Design review of the part shown in the three views and the two pictorial views. Dimensions are in mm from the part's minimum x, y and z. A direction names the side the tool comes from. Give positions to 0.01 mm unless a question says otherwise; leave off trailing zeros. Order: outer loops, then holes, each group sorted by start corner. A loop starts at its lowest first (then second) coordinate and runs counter-clockwise, first axis right, second up.
Item 1: The part is to be moulded in two halves that separate along X. For the marked faces 1, 2 and 3, say which applies: released by +X, released by -X, zero draft, split by the parting line, or undercut.
Item 2: For P1, Ø1.5, axis at x = 14, z = 1, coming from the +Y side, flat-tipped, find the tip position at first contact; note if it passes through.
Item 3: Machinability: for the marked faces 4, 5 and 6, which of the approach directions +Z, -Z, +X, -X, +Y, -Y give a long, thin tool a straight path to every point of the face, cutting with its end or side? Answer none if there is none.
Item 4: Consider section D-D (y = 7.75). Give the boundary of the cut face in (x, z), plus the area to 3 significant figures.
Item 5: Consider section A-A (y = 16.5). Give the boundary of the cut face in (x, z), plus the area to 3 significant figures.
Item 6: Consider section B-B (x = 7.6). Give the boundary of the cut face in (y, z), plus the area to 3 significant figures.
Item 7: For probe 1 along Y at (x, z) = (7.6, 0.95); probe 2 along X at (y, z) = (10.5, 0.85); probe 3 along Y at (x, z) = (14, 2.65), list the stretches that pass through material, from the lowest coordinate up.
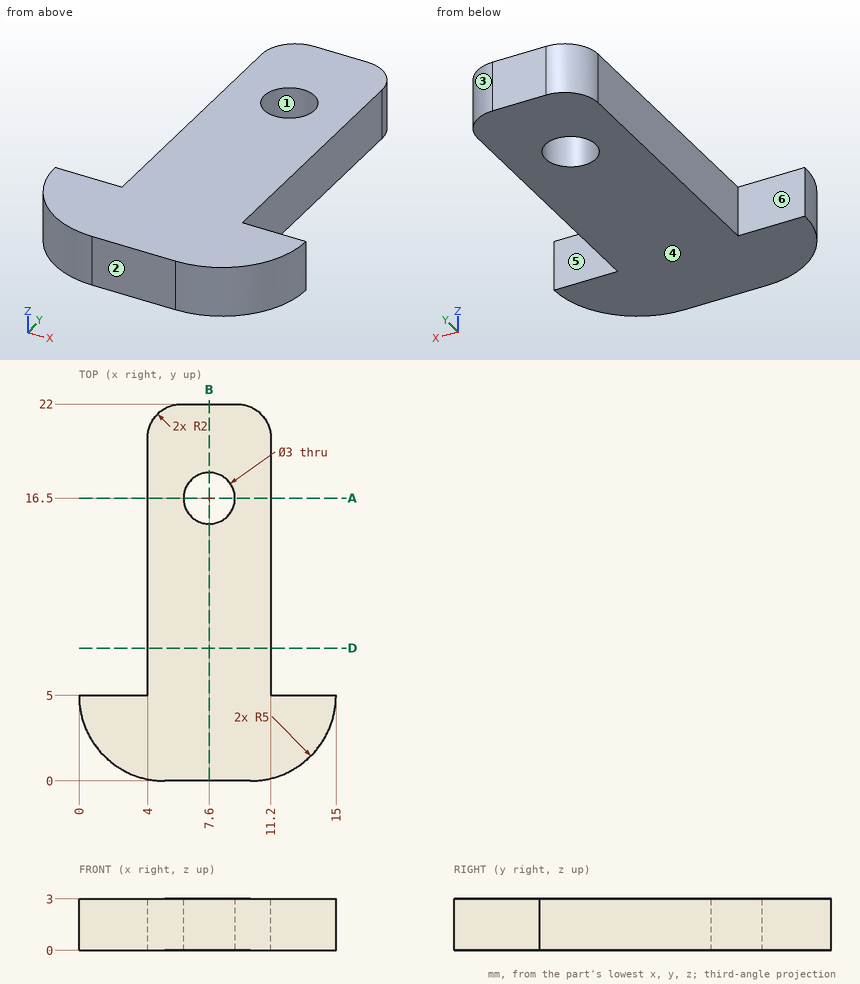
Resolved:
1. face 1: undercut
1. face 2: zero draft
1. face 3: released by +X
2. P1: stops at y = 5
3. face 4: -Z, +X, -X, +Y, -Y
3. face 5: +Z, -Z, +X, +Y
3. face 6: +Z, -Z, -X, +Y
4. outline: (4, 0) - (11.2, 0) - (11.2, 3) - (4, 3) - close
4. area: 21.6 mm2
5. outline: (4, 0) - (6.1, 0) - (6.1, 3) - (4, 3) - close; (9.1, 0) - (11.2, 0) - (11.2, 3) - (9.1, 3) - close
5. area: 12.6 mm2
6. outline: (0, 0) - (15, 0) - (15, 3) - (0, 3) - close; (18, 0) - (22, 0) - (22, 3) - (18, 3) - close
6. area: 57.0 mm2
7. probe 1: y = 0 to 15, 18 to 22
7. probe 2: x = 4 to 11.2
7. probe 3: y = 2 to 5
